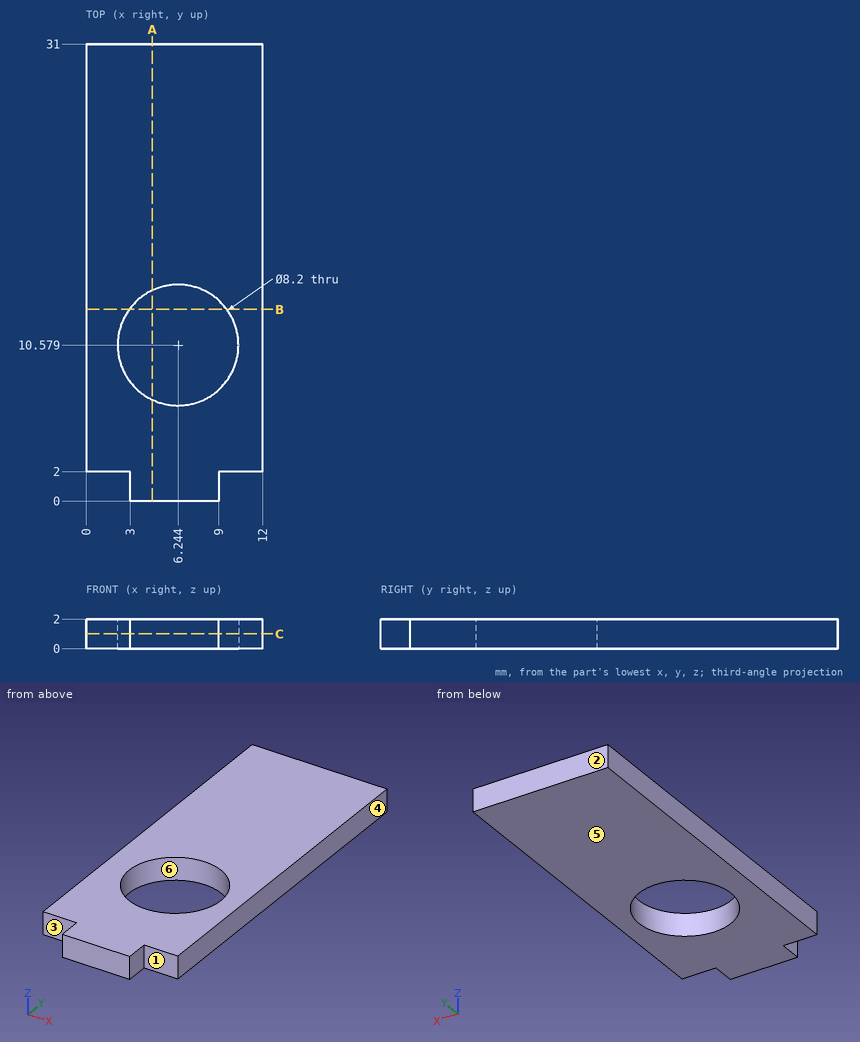
Input: dimensioned drawing with shaded views. Units: mm. Origin: part minimum x, y, z. A direction names the side the tool comes from. Round coordinates to 2 decimals unless told otherwise and drop trailing zeros. Loops run counter-clockwise (first coordinate to the right, second up) from the corner with the lowest first, then second, coordinate; pieces in that order, holes last. Notation, with made-up numbers: M 2.5,52.25 L 30.5,52.25 A23 ccw 30.5,66.25 Z; hole C 18.25,0.5 d10. An arc over 180 degrees is marked long. Return JSON: item names as keys, results as strings. Group by question number.
1. Reachability of the marked faces 1, 2 and 3 from +Z, -Z, +X, -X, +Y, -Y: full face, straight path, thin tool, end or side. Return the list, or none.
2. Section query A-A on x = 4.5. Output: boundary loops of the cut face in (y, z).
3. Section query C-C on z = 1. Output: boundary loops of the cut face in (x, y).
4. Pin query (flat end, axial travel): pin 1 (1 mm diameter, centred on x = 2, z = 0.5, fed in from -Y); pin 2 (0.6 mm diameter, centred on y = 1, z = 0.5, fed in from -X). Return the tip coordinate at first contact, or that it passes through.
5. Material intervals for line 1 along Y through (x, z) = (10, 1.3) (1 decimal); line 2 along Y through (x, z) = (4.5, 1); line 3 along X through (y, z) = (13.5, 0.4) (1 decimal), sorted ascending. Write a range as from..to.
6. Mould query, pull axis X, two halves, no side actions, for the marked faces 4, 5 and 6. Classes: released by +X, released by -X, zero draft, split by the parting line, or undercut.
7. Section query B-B on y = 13. Output: boundary loops of the cut face in (x, z) (1 decimal).
Checks:
{
 "1": {"face 1": "+Z, -Z, +X, -Y", "face 2": "+Z, -Z, +X, -X, +Y", "face 3": "+Z, -Z, -X, -Y"},
 "2": {"outline": "M 0,0 L 6.87,0 L 6.87,2 L 0,2 Z; M 14.29,0 L 31,0 L 31,2 L 14.29,2 Z"},
 "3": {"outline": "M 0,2 L 3,2 L 3,0 L 9,0 L 9,2 L 12,2 L 12,31 L 0,31 Z; hole C 6.24,10.58 d8.2"},
 "4": {"pin 1": "stops at y = 2", "pin 2": "stops at x = 3"},
 "5": {"line 1": "y = 2..8.9, 12.2..31", "line 2": "y = 0..6.87, 14.29..31", "line 3": "x = 0..3.4, 9.1..12"},
 "6": {"face 4": "released by +X", "face 5": "zero draft", "face 6": "undercut"},
 "7": {"outline": "M 0,0 L 2.9,0 L 2.9,2 L 0,2 Z; M 9.6,0 L 12,0 L 12,2 L 9.6,2 Z"}
}
